Study the drawing (mm; zero at the part's minimum x, y, z) and answer. A direction names the side the tool comes from. Coordinates: 2 decimals unless noted, no trailing zeros. Loops run counter-clockwise (first coordinate to the right, second up) from the corner with the lowest first, then second, coordinate; pieces in that order, holes last. Notation, with made-up numbers: (-15.5, 11) - (19.5, 11) arc R28 cw to (19.5, 41) - close; hole circle Ø1 at (19.25, -7.5). An arc over 180 degrees is marked (long way). Put each result on its own line as item: value.
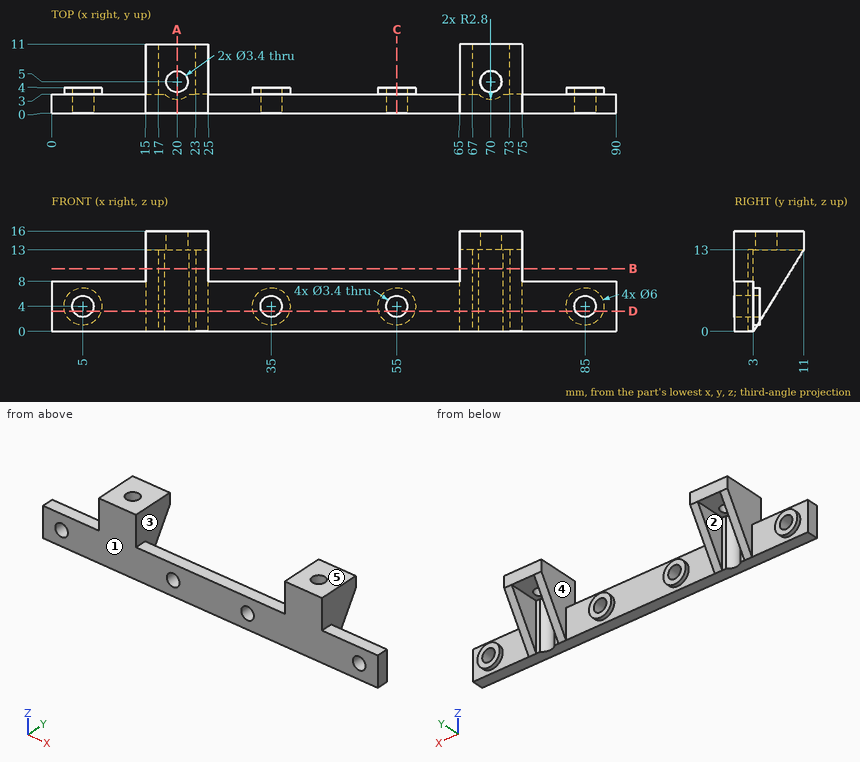
1) For the marked faces 1, 2 and 3, determine the directions among +Z, -Z, +X, -X, +Y, -Y from which every point of the face is accessible in a straight line to the end or side of a thin tool.
Found:
face 1: +Z, -Z, +X, -X, -Y
face 2: -Z, +Y
face 3: +Z, +Y
2) The part is cut by section D-D (z = 3.25). State how many separate pieces and enclosed holes the cut face has, and give its area (3 significant figures).
Found:
separate pieces: 5
enclosed holes: 0
area: 256 mm^2
3) For a pull along X with two mould halves and no side action, classify the marked faces 4 and 5 as pulls with the +X half, pulls with the -X half, needs draft (parallel to the pull), parting line crosses it, or undercut.
Found:
face 4: undercut
face 5: needs draft
4) Each of these flat-tipped pins is pushed along its axis until it touches: pin 1 (4.5 mm diameter, centred on x = 55, z = 4, fed in from -Y); pin 2 (3 mm diameter, centred on x = 71, y = 5, fed in from -Z); pin 3 (4 mm diameter, centred on y = 7.5, z = 8, fed in from -X); pin 4 (2.5 mm diameter, centred on x = 5, y = 1.5, fed in from +Z). Where does it stop, or does it pass through?
Found:
pin 1: stops at y = 0
pin 2: stops at z = 13
pin 3: stops at x = 15
pin 4: stops at z = 8
5) The part is cut by section A-A (x = 20). Give the vertices of the cut face in (y, z), and give its area (3 significant figures).
Found:
outline: (0, 0) - (2.2, 0) - (2.2, 13) - (3.3, 13) - (3.3, 16) - (0, 16) - close; (6.7, 13) - (11, 13) - (11, 16) - (6.7, 16) - close
area: 51.4 mm^2
6) The part is cut by section B-B (z = 10). Give the vertices of the cut face in (x, y), and give its area (3 significant figures).
Found:
outline: (15, 0) - (25, 0) - (25, 9.15) - (23, 9.15) - (23, 3) - (21.96, 3) arc R2.8 cw to (18.04, 3) - (17, 3) - (17, 9.15) - (15, 9.15) - close; (65, 0) - (75, 0) - (75, 9.15) - (73, 9.15) - (73, 3) - (71.96, 3) arc R2.8 cw to (68.04, 3) - (67, 3) - (67, 9.15) - (65, 9.15) - close
area: 105 mm^2
7) Straight lines are drawn through the part: L1, parallel to X at y = 1.3, z = 4; L2, parallel to X at y = 5.75, z = 12; L3, parallel to Y at x = 20, z = 15.4. For each, find the intervals that lie inside material, in ascending order. Write a range as [from, to].
Found:
L1: x = [0, 3.3], [6.7, 33.3], [36.7, 53.3], [56.7, 83.3], [86.7, 90]
L2: x = [15, 17], [23, 25], [65, 67], [73, 75]
L3: y = [0, 3.3], [6.7, 11]
8) The part is cut by section C-C (x = 55). Give the vertices of the cut face in (y, z).
Found:
outline: (0, 0) - (3, 0) - (3, 1) - (4, 1) - (4, 2.3) - (0, 2.3) - close; (0, 5.7) - (4, 5.7) - (4, 7) - (3, 7) - (3, 8) - (0, 8) - close
